```python
from build123d import *

# Parameters (mm, degrees)
SKETCH1_W           = 160
SKETCH1_H           = 135
BOSS_EXTRUDE1_DEPTH = 3
CUT_EXTRUDE1_DEPTH  = 20


with BuildPart() as part:
    # Sketch1 → Boss-Extrude1 (new body)
    with BuildSketch(Plane.XY.offset(152)):
        with Locations((0, 12.91714511)):
            Rectangle(SKETCH1_W, SKETCH1_H)
        with BuildLine():
            Line((-60, -22.204596664), (-60, 48.038886885))
            ThreePointArc((-60, 48.038886885), (-56.872665603, 52.674954566), (-51.402750584, 51.511608676))
            Line((-51.402750584, 51.511608676), (-17.49683417, 16.389866902))
            ThreePointArc((-17.49683417, 16.389866902), (-16.094083586, 12.91714511), (-17.49683417, 9.444423319))
            Line((-17.49683417, 9.444423319), (-51.402750584, -25.677318456))
            ThreePointArc((-51.402750584, -25.677318456), (-56.872665603, -26.840664345), (-60, -22.204596664))
        make_face(mode=Mode.SUBTRACT)
        with BuildLine():
            Line((20.424315219, 60.41714511), (-20.424315219, 60.41714511))
            ThreePointArc((-20.424315219, 60.41714511), (-25.026684661, 57.371165459), (-24.021564635, 51.944423319))
            Line((-24.021564635, 51.944423319), (-3.597249416, 30.787716735))
            ThreePointArc((-3.597249416, 30.787716735), (0, 29.260438526), (3.597249416, 30.787716735))
            Line((3.597249416, 30.787716735), (24.021564635, 51.944423319))
            ThreePointArc((24.021564635, 51.944423319), (25.026684661, 57.371165459), (20.424315219, 60.41714511))
        make_face(mode=Mode.SUBTRACT)
        with BuildLine():
            Line((51.402750584, 51.511608676), (17.49683417, 16.389866902))
            ThreePointArc((17.49683417, 16.389866902), (16.094083586, 12.91714511), (17.49683417, 9.444423319))
            Line((17.49683417, 9.444423319), (51.402750584, -25.677318456))
            ThreePointArc((51.402750584, -25.677318456), (56.872665603, -26.840664345), (60, -22.204596664))
            Line((60, -22.204596664), (60, 48.038886885))
            ThreePointArc((60, 48.038886885), (56.872665603, 52.674954566), (51.402750584, 51.511608676))
        make_face(mode=Mode.SUBTRACT)
        with BuildLine():
            Line((-24.021564635, -26.110133098), (-3.597249416, -4.953426514))
            ThreePointArc((-3.597249416, -4.953426514), (0, -3.426148305), (3.597249416, -4.953426514))
            Line((3.597249416, -4.953426514), (24.021564635, -26.110133098))
            ThreePointArc((24.021564635, -26.110133098), (25.026684661, -31.536875238), (20.424315219, -34.58285489))
            Line((20.424315219, -34.58285489), (-20.424315219, -34.58285489))
            ThreePointArc((-20.424315219, -34.58285489), (-25.026684661, -31.536875238), (-24.021564635, -26.110133098))
        make_face(mode=Mode.SUBTRACT)
    extrude(amount=BOSS_EXTRUDE1_DEPTH)

    # Sketch2 → Cut-Extrude1 (cut)
    with BuildSketch(Plane.XY.offset(155)):
        with BuildLine():
            ThreePointArc((1.5, -41.631936217), (0, -40.131936217), (-1.5, -41.631936217))
            Line((-1.5, -41.631936217), (1.5, -41.631936217))
        make_face()
        with BuildLine():
            Line((1.5, -41.631936217), (-1.5, -41.631936217))
            ThreePointArc((-1.5, -41.631936217), (0, -43.131936217), (1.5, -41.631936217))
        make_face()
    extrude(amount=-CUT_EXTRUDE1_DEPTH, mode=Mode.SUBTRACT)


solid = part.part
```
Here's how the part is built. I have some questions about the finished solid (model axes, mm). A direction names the side the tool comes from. Give positions to 0.01 mm unless a question says otherwise; leave off trailing zeros. Order: outer loops, then holes, each group sorted by start corner. A loop starts at its lowest first (then second) coordinate and runs counter-clockwise, first axis right, second up. Notation, with made-up numbers: (73, 23.5) -> (126, 23.5) arc R18 ccw to (126, 45.5) -> close; hole circle Ø1 at (55, 22). An arc over 180 degrees is marked (long way). Use CSV: the item, a comma, the result in double quotes. Start each with the question number.
Item 1: Suppose I cut it at C-C (x = 11). List the corners of the cut face in (y, z) for me.
Item 2: Suppose I cut it at A-A (y = 45). List the corners of the cut face in (x, z) for me.
Item 3: On a 3-axis mill with a long thin cutter (end or side, diameter ignored), from which of +Z, -Z, +X, -X, +Y, -Y can I reach the whole of each face in a straight line? I mean faces 1 (the cylindrical face through (56.949, 52.643, 153.479)), 2 (the flat face through (-1, 14, 152)). Say none if no direction works.
Item 4: If I drill on probe 1 along Y at (x, z) = (0, 153.9); probe 2 along Y at (x, z) = (14, 153.95); probe 3 along X at (y, z) = (38.5, 152.25), over which ranges is the centre line in solid material (lowest first)? Write a range as [from, to].
Item 5: Suppose I cut it at D-D (y = 19.5). List the corners of the cut face in (x, z) for me, and give its area (3 significant figures).
Item 6: Thinking about a two-plate mould opening in X: for faces 3 (the flat face through (-13.95, 41.51, 153.48)), 4 (the flat face through (-1, 14, 155)), which applies, pulls with the +X half, pulls with the -X half, needs draft (parallel to the pull), parting line crosses it, or undercut?
Item 7: Suppose I cut it at B-B (x = -45). List the corners of the cut face in (y, z) for me, and give its area (3 significant figures).
Answer block:
1,outline,"(-54.58, 152) -> (-34.58, 152) -> (-34.58, 155) -> (-54.58, 155) -> close; (-12.62, 152) -> (38.46, 152) -> (38.46, 155) -> (-12.62, 155) -> close; (60.42, 152) -> (80.42, 152) -> (80.42, 155) -> (60.42, 155) -> close"
2,outline,"(-80, 152) -> (-60, 152) -> (-60, 155) -> (-80, 155) -> close; (-45.12, 152) -> (-17.32, 152) -> (-17.32, 155) -> (-45.12, 155) -> close; (17.32, 152) -> (45.12, 152) -> (45.12, 155) -> (17.32, 155) -> close; (60, 152) -> (80, 152) -> (80, 155) -> (60, 155) -> close"
3,face 1,"+Z, -Z"
3,face 2,"-Z, +X, -X, +Y, -Y"
4,probe 1,"y = [-54.58, -43.13], [-40.13, -34.58], [-3.43, 29.26], [60.42, 80.42]"
4,probe 2,"y = [-54.58, -34.58], [-15.73, 41.56], [60.42, 80.42]"
4,probe 3,"x = [-80, -60], [-38.84, -11.04], [11.04, 38.84], [60, 80]"
5,outline,"(-80, 152) -> (-60, 152) -> (-60, 155) -> (-80, 155) -> close; (-20.5, 152) -> (20.5, 152) -> (20.5, 155) -> (-20.5, 155) -> close; (60, 152) -> (80, 152) -> (80, 155) -> (60, 155) -> close"
5,area,"243 mm^2"
6,face 3,"undercut"
6,face 4,"needs draft"
7,outline,"(-54.58, 152) -> (-19.04, 152) -> (-19.04, 155) -> (-54.58, 155) -> close; (44.88, 152) -> (80.42, 152) -> (80.42, 155) -> (44.88, 155) -> close"
7,area,"213 mm^2"
